from build123d import *

# Parameters (mm, degrees)
F0_W     = 26
F0_H     = 10
F1_DEPTH = 30
F2_W     = 26
F2_H     = 10
F2_W_2   = 24
F2_H_2   = 8
F3_DEPTH = 1
F5_DEPTH = 2


with BuildPart() as f1:
    # F0 (on Top) → F1 (new body)
    with BuildSketch(Plane.XY):
        Rectangle(F0_W, F0_H)
    extrude(amount=F1_DEPTH)

    # F2 (on face) → F3 (join)
    with BuildSketch(Plane(origin=(0, 0, 0), x_dir=(1, 0, 0), z_dir=(0, 0, -1))):
        Rectangle(F2_W, F2_H)
        Rectangle(F2_W_2, F2_H_2, mode=Mode.SUBTRACT)
    extrude(amount=F3_DEPTH)

    # F4 (on face) → F5 (join)
    with BuildSketch(Plane.XZ.offset(5)):
        with BuildLine():
            Line((-3, 27), (-9, 27))
            Line((-9, 27), (-9, 2))
            Line((-9, 2), (-3, 2))
            Line((-3, 2), (-3, 10))
            Line((-3, 10), (0.5, 10))
            ThreePointArc((0.5, 10), (9, 18.5), (0.5, 27))
            Line((0.5, 27), (-3, 27))
        make_face()
        with BuildLine():
            Line((-3, 16), (-3, 21))
            Line((-3, 21), (0.5, 21))
            ThreePointArc((0.5, 21), (3, 18.5), (0.5, 16))
            Line((0.5, 16), (-3, 16))
        make_face(mode=Mode.SUBTRACT)
    extrude(amount=F5_DEPTH)


solid = f1.part
Could you check a few things on this model? Use its own coordinates, in mm. A direction names the side the tool comes from. Round coordinates to 2 decimals unless told otherwise and drop trailing zeros. Order: outer loops, then holes, each group sorted by start corner. A loop starts at its lowest first (then second) coordinate and runs counter-clockwise, first axis right, second up.
(1) Imagine slicing it at B-B (z = 18.5). Write out the boundary of the cut face in (x, y).
Response values:
outline: (-13, -5) - (-9, -5) - (-9, -7) - (-3, -7) - (-3, -5) - (3, -5) - (3, -7) - (9, -7) - (9, -5) - (13, -5) - (13, 5) - (-13, 5) - close
(2) Imagine slicing it at D-D (z = 14.5). Write out the boundary of the cut face in (x, y).
Response values:
outline: (-13, -5) - (-9, -5) - (-9, -7) - (8, -7) - (8, -5) - (13, -5) - (13, 5) - (-13, 5) - close
(3) Which directions (+Z, -Z, +X, -X, +Y, -Y) give clear straight access to the entire face, cutting with the end or side of a thin tool? Please do faces 4 (the flat face through (-6, -6, 2)), 5 (the flat face through (-4, -6, 27)), 6 (the flat face through (-1, -6, 10)), 7 (the flat face through (-12, 0.1, -0.5)), 8 (the flat face through (0, -5, 19)).
Response values:
face 4: -Z, +X, -X, -Y
face 5: +Z, +X, -X, -Y
face 6: -Z, +X, -Y
face 7: -Z
face 8: -Y
(4) Imagine slicing it at C-C (x = -4). Write out the boundary of the cut face in (y, z), plus the area to 3 significant figures.
Response values:
outline: (-7, 2) - (-5, 2) - (-5, -1) - (-4, -1) - (-4, 0) - (4, 0) - (4, -1) - (5, -1) - (5, 30) - (-5, 30) - (-5, 27) - (-7, 27) - close
area: 352 mm2
(5) If we mould it in two halves opening along Y, with no side actions, what happens to faces 1 (the flat face through (-2, -7, 15)), 2 (the flat face through (13, 0, 15)), 3 (the flat face through (-0.2, 4, -0.5))? For each: released by +Y, released by -Y, zero draft, split by the parting line, or undercut.
Response values:
face 1: released by -Y
face 2: zero draft
face 3: undercut
(6) I'm going to push flat-ended pins straight in: pin 1 (2 mm diameter, centred on x = 5.5, y = -0.5, fed in from -Z); pin 2 (5.5 mm diameter, centred on x = 0, z = 17.5, fed in from -Y); pin 3 (0.6 mm diameter, centred on y = -6.5, z = 19, fed in from +X); pin 4 (1.6 mm diameter, centred on x = -5.5, y = -6.5, fed in from -Z). Where does each tip first touch, or does it pass through?
Response values:
pin 1: stops at z = 0
pin 2: stops at y = -7
pin 3: stops at x = 9
pin 4: stops at z = 2
(7) Please list where these lines run through material, in increasing order: line 1 along Z through (x, y) = (-1, -5.25); line 2 along Y through (x, z) = (8.75, 21.5); line 3 along Z through (x, y) = (7, 2.25).
Response values:
line 1: z = 10 to 16, 21 to 27
line 2: y = -5 to 5
line 3: z = 0 to 30
(8) Imagine slicing it at A-A (y = 0.25). Write out the boundary of the cut face in (x, z).
Response values:
outline: (-13, -1) - (-12, -1) - (-12, 0) - (12, 0) - (12, -1) - (13, -1) - (13, 30) - (-13, 30) - close
